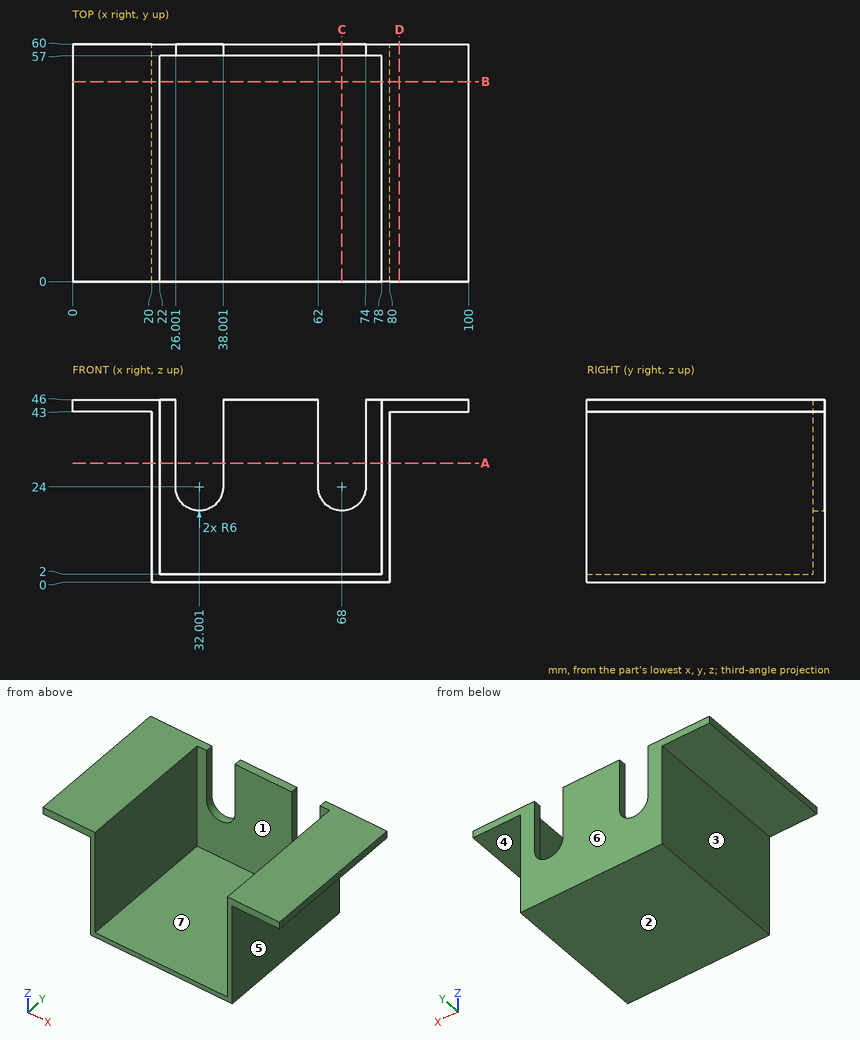
Here's the drawing with two shaded views (mm, measured from the low corner). I have some questions. A direction names the side the tool comes from. Round coordinates to 2 decimals unless told otherwise and drop trailing zeros. Order: outer loops, then holes, each group sorted by start corner. A loop starts at its lowest first (then second) coordinate and runs counter-clockwise, first axis right, second up. Notation, with made-up numbers: (14.5, -26) -> (41.5, -26) arc R23 ccw to (41.5, -10) -> close; hole circle Ø5 at (59, -31). An arc over 180 degrees is marked (long way). Return JSON: item names as keys, results as strings.
Q1. If we mould it in two halves opening along X, with no side actions, what happens to the marked faces 5, 6 and 7? For each: released by +X, released by -X, zero draft, split by the parting line, or undercut.
Filled sheet:
{"face 5": "released by +X", "face 6": "zero draft", "face 7": "undercut"}
Q2. If we section it at B-B on y = 50.5: List the corners of the cut face in (x, z) for me, plus the area to 3 significant figures.
Filled sheet:
{"outline": "(0, 43) -> (20, 43) -> (20, 0) -> (80, 0) -> (80, 43) -> (100, 43) -> (100, 46) -> (78, 46) -> (78, 2) -> (22, 2) -> (22, 46) -> (0, 46) -> close", "area": "416 mm^2"}
Q3. I need wall thicknesses on line 1 along X through (y, z) = (32, 34.5); line 2 along Y through (x, z) = (55, 26.5); line 3 along Z through (x, y) = (23, 14). Which ranges of each line are inside material? Lowest first, please. Write a range as from..to.
Filled sheet:
{"line 1": "x = 20..22, 78..80", "line 2": "y = 57..60", "line 3": "z = 0..2"}
Q4. If we section it at A-A on z = 30: List the corners of the cut face in (x, y) for me, plus the area to 3 significant figures.
Filled sheet:
{"outline": "(20, 0) -> (22, 0) -> (22, 57) -> (26, 57) -> (26, 60) -> (20, 60) -> close; (38, 57) -> (62, 57) -> (62, 60) -> (38, 60) -> close; (74, 57) -> (78, 57) -> (78, 0) -> (80, 0) -> (80, 60) -> (74, 60) -> close", "area": "336 mm^2"}
Q5. For pin 1 Ø2.5 at (y, z) = (59, 37.5) entering from -X; pin 2 Ø8 at (x, z) = (87, 10.5) entering from -Y; pin 3 Ø21.5 at (y, z) = (25.5, 31) entering from +X; pin 4 Ø10 at (x, y) = (12.5, 24) entering from -Z, each with a flat end and sliding along its axis, tell me the tip position at first contact or that it passes through.
Filled sheet:
{"pin 1": "stops at x = 20", "pin 2": "passes through", "pin 3": "stops at x = 80", "pin 4": "stops at z = 43"}
Q6. Which directions (+Z, -Z, +X, -X, +Y, -Y) give clear straight access to the entire face, cutting with the end or side of a thin tool? Please do the marked faces 1, 2, 3 and 4.
Filled sheet:
{"face 1": "+Z, -Y", "face 2": "-Z, +X, -X, +Y, -Y", "face 3": "-Z, -X, +Y, -Y", "face 4": "-Z, +X, +Y, -Y"}
Q7. If we section it at D-D on x = 82.5: List the corners of the cut face in (y, z) for me.
Filled sheet:
{"outline": "(0, 43) -> (60, 43) -> (60, 46) -> (0, 46) -> close"}
Q8. If we section it at C-C on x = 68: List the corners of the cut face in (y, z) for me, plus the area to 3 significant figures.
Filled sheet:
{"outline": "(0, 0) -> (60, 0) -> (60, 18) -> (57, 18) -> (57, 2) -> (0, 2) -> close", "area": "168 mm^2"}
